```python
from build123d import *

# Parameters (mm, degrees)
F0_W     = 152.4
F0_H     = 76.2
F1_DEPTH = 25.4
F2_W     = 139.7
F2_H     = 50.8
F3_DEPTH = 19.05
F4_W     = 6.35
F4_H     = 11.1125
F5_DEPTH = 139.7
F6_R     = 1.7018
F7_DEPTH = 12.7


with BuildPart() as f1:
    # F0 (on Top) → F1 (new body)
    with BuildSketch(Plane.XY):
        Rectangle(F0_W, F0_H)
    extrude(amount=F1_DEPTH)

    # F2 (on face) → F3 (cut)
    with BuildSketch(Plane.XY.offset(25.4)):
        with Locations((-6.35, 0)):
            Rectangle(F2_W, F2_H)
    extrude(amount=-F3_DEPTH, mode=Mode.SUBTRACT)

    # F4 (on face) → F5 (cut)
    with BuildSketch(Plane(origin=(-76.2, 0, 0), x_dir=(0, -1, 0), z_dir=(-1, 0, 0))):
        with Locations((-28.575, 11.90625)):
            Rectangle(F4_W, F4_H)
        with Locations((28.575, 11.90625)):
            Rectangle(F4_W, F4_H)
    extrude(amount=-F5_DEPTH, mode=Mode.SUBTRACT)

    # F6 (on face) → F7 (cut)
    with BuildSketch(Plane(origin=(63.5, 0, 0), x_dir=(0, -1, 0), z_dir=(-1, 0, 0))):
        with Locations((0, 12.7)):
            Circle(F6_R)
    extrude(amount=-F7_DEPTH, mode=Mode.SUBTRACT)


solid = f1.part
```
Can you work these out from the model? Positions are in its coordinate system, mm. A direction names the side the tool comes from. Coordinates: 2 decimals unless noted, no trailing zeros. Loops run counter-clockwise (first coordinate to the right, second up) from the corner with the lowest first, then second, coordinate; pieces in that order, holes last.
Item 1: Suppose I cut it at A-A (y = 0). Please give me the cut outline in (x, z).
Answers below:
outline: (-76.2, 0) - (76.2, 0) - (76.2, 11) - (63.5, 11) - (63.5, 6.35) - (-76.2, 6.35) - close; (63.5, 14.4) - (76.2, 14.4) - (76.2, 25.4) - (63.5, 25.4) - close
Item 2: Suppose I cut it at B-B (z = 12.7). Please give me the cut outline in (x, y).
Answers below:
outline: (-76.2, -38.1) - (76.2, -38.1) - (76.2, -1.7) - (63.5, -1.7) - (63.5, -31.75) - (-76.2, -31.75) - close; (-76.2, 31.75) - (63.5, 31.75) - (63.5, 1.7) - (76.2, 1.7) - (76.2, 38.1) - (-76.2, 38.1) - close
Item 3: Which directions (+Z, -Z, +X, -X, +Y, -Y) give clear straight access to the entire face, cutting with the end or side of a thin tool? Please do faces 5 (the face through (-7, 29, 17.462)), 6 (the face through (-7, 25.4, 21)), 7 (the face through (16, 26, 25.4)).
Answers below:
face 5: -X
face 6: +Z, -X
face 7: +Z, +X, -X, +Y, -Y
Item 4: Suppose I cut it at D-D (x = 50). Please give me the cut outline in (y, z), then the cut area to 3 significant figures.
Answers below:
outline: (-38.1, 0) - (38.1, 0) - (38.1, 25.4) - (25.4, 25.4) - (25.4, 17.46) - (31.75, 17.46) - (31.75, 6.35) - (-31.75, 6.35) - (-31.75, 17.46) - (-25.4, 17.46) - (-25.4, 25.4) - (-38.1, 25.4) - close
area: 827 mm2
Item 5: If we mould it in two halves opening along Y, with no side actions, what happens to faces 1 (the face through (-1, -38.1, 13)), 2 (the face through (63.5, 0, 16)), 3 (the face through (-1, 38.1, 13)), 4 (the face through (76.2, -1, 15))? For each: released by +Y, released by -Y, zero draft, split by the parting line, or undercut.
Answers below:
face 1: released by -Y
face 2: undercut
face 3: released by +Y
face 4: zero draft
Item 6: Please list where these lines run through material, in increasing order: L1, parallel to Z at x = 68.5, y = 0; L2, parallel to Y at x = -17, z = 23.75; L3, parallel to Y at x = 50.5, z = 12.5.
Answers below:
L1: z = 0 to 11, 14.4 to 25.4
L2: y = -38.1 to -25.4, 25.4 to 38.1
L3: y = -38.1 to -31.75, 31.75 to 38.1
Item 7: Suppose I cut it at C-C (y = 28.5). Please give me the cut outline in (x, z), then the cut area to 3 significant figures.
Answers below:
outline: (-76.2, 0) - (76.2, 0) - (76.2, 25.4) - (-76.2, 25.4) - (-76.2, 17.46) - (63.5, 17.46) - (63.5, 6.35) - (-76.2, 6.35) - close
area: 2,320 mm2
Item 8: I'm going to push flat-ended pins straight in: pin 1 (4 mm diameter, centred on x = 49, y = 28.5, fed in from -Z); pin 2 (6 mm diameter, centred on y = -9.5, z = 17, fed in from -X). Where does each tip first touch, or does it pass through?
Answers below:
pin 1: stops at z = 0
pin 2: stops at x = 63.5
